```python
from build123d import *

# Parameters (mm, degrees)
SKICA1_W                = 57
SKICA1_H                = 67
SKICA1_R                = 2
P_IDAT_VYSUNUT_M1_DEPTH = 3
P_IDAT_VYSUNUT_M2_DEPTH = 1
ZAOBLIT1_R              = 3


with BuildPart() as part:
    # Skica1 → Přidat vysunutím1 (new body)
    with BuildSketch(Plane.XY):
        with Locations((28.5, 33.5)):
            Rectangle(SKICA1_W, SKICA1_H)
        with Locations((3.5, 62.35016579)):
            Circle(SKICA1_R, mode=Mode.SUBTRACT)
        with Locations((53.5, 62.35016579)):
            Circle(SKICA1_R, mode=Mode.SUBTRACT)
        with Locations((53.5, 3.5)):
            Circle(SKICA1_R, mode=Mode.SUBTRACT)
        with Locations((3.5, 3.5)):
            Circle(SKICA1_R, mode=Mode.SUBTRACT)
    extrude(amount=P_IDAT_VYSUNUT_M1_DEPTH)

    # Skica2 → Přidat vysunutím2 (add)
    with BuildSketch(Plane(origin=(0, 0, 0), x_dir=(-1, 0, 0), z_dir=(0, 0, -1))):
        Polygon((-41.396588298, 31.388427372), (-41.396588298, 33.183299167), (-23.447870349, 33.183299167), (-23.447870349, 40.87560686), (-21.396588298, 40.87560686), (-21.396588298, 31.388427372), align=None)
    extrude(amount=P_IDAT_VYSUNUT_M2_DEPTH)

    # Zaoblit1
    zaoblit1_edges = [part.edges().sort_by_distance(p)[0] for p in [
        (0, 67, 1.5),
        (57, 67, 1.5),
        (57, 0, 1.5),
        (0, 0, 1.5),
    ]]
    fillet(zaoblit1_edges, radius=ZAOBLIT1_R)


solid = part.part
```
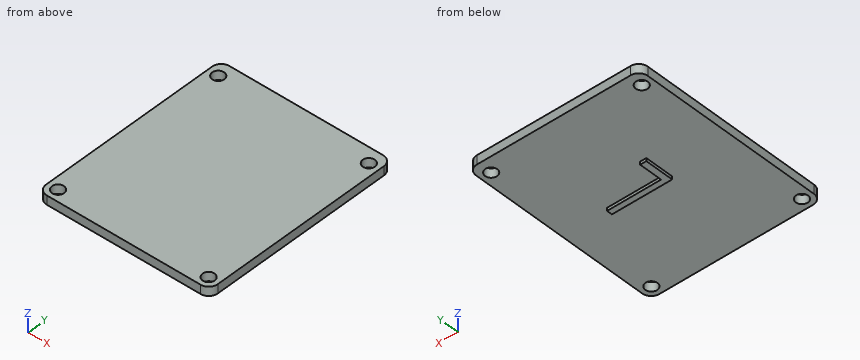
Design review of the part built by this model. Coordinates are the model's own, in mm. Give positions to 0.01 mm unless a question says otherwise; leave off trailing zeros. Loops run counter-clockwise (first coordinate to the right, second up) from the corner with the lowest first, then second, coordinate; pieces in that order, holes last. Notation, with made-up numbers: M 64.25,36 L 71.25,36 A30 ccw 71.25,60 Z; hole C 77.5,71 d3. An arc over 180 degrees is marked long. Return JSON: item names as keys, results as strings. Group by question number.
Item 1: For probe 1 along Y at (x, z) = (53.5, 1.8); probe 2 along X at (y, z) = (4.5, 0.1); probe 3 along Z at (x, y) = (11, 55.5), list the stretches that pass through material, from the lowest coordinate up.
Item 2: We need section D-D (x = 11). Give the boundary of the cut face in (y, z).
Item 3: We need section C-C (y = 47). Give the boundary of the cut face in (x, z).
Item 4: Insertion check: pin 1 Ø2.5 at (x, y) = (3.5, 3.5) entering from +Z; pin 2 Ø12 at (x, y) = (39, 23) entering from -Z; pin 3 Ø0.5 at (x, z) = (22, -0.5) entering from +Y; pin 4 Ø0.8 at (x, z) = (31, -0.5) entering from -Y. Each pin has a flat end and moves straight along its axis. Give the tip position at first contact, or say it passes through.
Item 5: We need section A-A (x = 34). Give the boundary of the cut face in (y, z).
Item 6: We need section B-B (z = 1.7). Give the boundary of the cut face in (x, y), and give its area (3 significant figures).
Output:
{
 "1": {"probe 1": "y = 0 to 1.5, 5.5 to 60.35, 64.35 to 67", "probe 2": "x = 0 to 1.77, 5.23 to 51.77, 55.23 to 57", "probe 3": "z = 0 to 3"},
 "2": {"outline": "M 0,0 L 67,0 L 67,3 L 0,3 Z"},
 "3": {"outline": "M 0,0 L 57,0 L 57,3 L 0,3 Z"},
 "4": {"pin 1": "passes through", "pin 2": "stops at z = 0", "pin 3": "stops at y = 40.88", "pin 4": "stops at y = 31.39"},
 "5": {"outline": "M 0,0 L 31.39,0 L 31.39,-1 L 33.18,-1 L 33.18,0 L 67,0 L 67,3 L 0,3 Z"},
 "6": {"outline": "M 0,3 A3 ccw 3,0 L 54,0 A3 ccw 57,3 L 57,64 A3 ccw 54,67 L 3,67 A3 ccw 0,64 Z; hole C 3.5,3.5 d4; hole C 3.5,62.35 d4; hole C 53.5,3.5 d4; hole C 53.5,62.35 d4", "area": "3,760 mm^2"}
}
